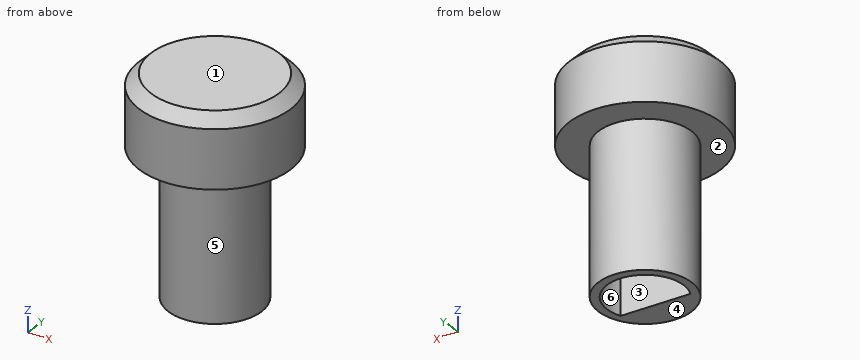
from build123d import *

# Parameters (mm, degrees)
SKETCH063_R     = 6.5
PAD036_DEPTH    = 6
CHAMFER002_SIZE = 1
SKETCH066_R     = 4
PAD038_DEPTH    = 12.5
POCKET030_DEPTH = 7


with BuildPart() as part:
    # Sketch063 → Pad036 (new body)
    with BuildSketch(Plane(origin=(0, 0, 30), x_dir=(1, 0, 0), z_dir=(0, 0, -1))):
        with Locations((14.5, -4)):
            Circle(SKETCH063_R)
    extrude(amount=-PAD036_DEPTH)

    # Chamfer002
    chamfer002_edges = [part.edges().sort_by_distance(p)[0] for p in [
        (8, 4, 36),
    ]]
    chamfer(chamfer002_edges, length=CHAMFER002_SIZE)

    # Sketch066 (on Face3 of Chamfer002) → Pad038 (join)
    with BuildSketch(Plane(origin=(0, 0, 30), x_dir=(1, 0, 0), z_dir=(0, 0, -1))):
        with Locations((14.5, -4)):
            Circle(SKETCH066_R)
    extrude(amount=PAD038_DEPTH)

    # Sketch067 (on Face5 of Pad038) → Pocket030 (cut)
    with BuildSketch(Plane(origin=(0, 0, 17.5), x_dir=(1, 0, 0), z_dir=(0, 0, -1))):
        with BuildLine():
            ThreePointArc((11.5, -2.602698), (14.5, -7.263055), (17.5, -2.602698))
            Line((14.5, -2.602698), (17.5, -2.602698))
            Line((14.5, -2.602698), (11.5, -2.602698))
        make_face()
    extrude(amount=-POCKET030_DEPTH, mode=Mode.SUBTRACT)


with BuildPart() as part_1:
    # Body005 placement: moved
    add(part.part.moved(Location((0, 2, 2.5))))


solid = part_1.part
Verification items for the finished model (mm, model axes). Face numbers are marked on the shaded views. A direction names the side the tool comes from. Round coordinates to 2 decimals unless told otherwise and drop trailing zeros. Loops run counter-clockwise (first coordinate to the right, second up) from the corner with the lowest first, then second, coordinate; pieces in that order, holes last. Notation, with made-up numbers: (-6, 15) - (20, 15) arc R22 ccw to (20, 34) - close; hole circle Ø8 at (57.25, -39). An arc over 180 degrees is marked (long way). Use one line per item in the form item = value.
1. Scan lines: probe 1 along Y at (x, z) = (14.5, 22.25); probe 2 along Z at (x, y) = (14.25, 11); probe 3 along Y at (x, z) = (16.75, 25.25). Record each from-to range of solid material in increasing order.
A:
probe_1 = 2 to 4.6, 9.26 to 10
probe_2 = 32.5 to 38.5
probe_3 = 2.69 to 4.6, 8.38 to 9.31
2. Draft check along Y on the marked faces 3, 4, 5 and 6. Enter one of: pulls with the +Y half, pulls with the -Y half, needs draft (parallel to the pull), parting line crosses it, or undercut.
A:
face_3 = undercut
face_4 = needs draft
face_5 = parting line crosses it
face_6 = undercut
3. Section check C-C on z = 34.5. Record the cut outline in (x, y).
A:
outline = circle Ø13 at (14.5, 6)
4. Access from +Z, -Z, +X, -X, +Y, -Y to the whole of each face (thin tool, end or side, straight path). Record for the marked faces 1 and 2.
A:
face_1 = +Z, +X, -X, +Y, -Y
face_2 = -Z
5. Section check D-D on z = 31. Record the cut outline in (x, y), and give its area (3 significant figures).
A:
outline = circle Ø8 at (14.5, 6)
area = 50.3 mm²
6. Section check A-A on x = 14.5. Record the cut outline in (y, z), and give its area (3 significant figures).
A:
outline = (-0.5, 32.5) - (2, 32.5) - (2, 20) - (4.6, 20) - (4.6, 27) - (9.26, 27) - (9.26, 20) - (10, 20) - (10, 32.5) - (12.5, 32.5) - (12.5, 37.5) - (11.5, 38.5) - (0.5, 38.5) - (-0.5, 37.5) - close
area = 144 mm²
7. Section check B-B on y = 6. Record the cut outline in (x, z).
A:
outline = (8, 32.5) - (10.5, 32.5) - (10.5, 20) - (11.2, 20) - (11.2, 27) - (17.8, 27) - (17.8, 20) - (18.5, 20) - (18.5, 32.5) - (21, 32.5) - (21, 37.5) - (20, 38.5) - (9, 38.5) - (8, 37.5) - close
8. Gauge pin test, flat ends, axial feed: pin 1 Ø5 at (y, z) = (8, 23) entering from +X; pin 2 Ø1.5 at (x, z) = (18.5, 25.5) entering from -Y; pin 3 Ø6 at (x, z) = (9.5, 23.5) entering from -Y. Record the tip position at first contact, or that the pin passes through.
A:
pin_1 = 18.5
pin_2 = 3.67
pin_3 = 2.54
